Could you check a few things on this model? Use its own coordinates, in mm. A direction names the side the tool comes from. Round coordinates to 2 decimals unless told otherwise and drop trailing zeros. Loops run counter-clockwise (first coordinate to the right, second up) from the corner with the lowest first, then second, coordinate; pieces in that order, holes last. Notation, with made-up numbers: (-24, -33) - (-1, -33) arc R24 cw to (-1, -9) - close; hole circle Ø10 at (-18, 35). An arc over 180 degrees is marked (long way). Answer as CSV lines item,"result". Start each with the question number.
1) Which directions (+Z, -Z, +X, -X, +Y, -Y) give clear straight access to the entire face, cutting with the end or side of a thin tool? Please do faces 1 (the face through (25.5, 43, -63)), 2 (the face through (-20.5, -12, -58)), 3 (the face through (-28, -17.5, -10)), 4 (the face through (-30.3, 13.5, -17)).
2) We'd pull the mould along Z, two halves only. Please class faces 5 (the face through (0, 12, -34)), 6 (the face through (-6.5, 14, -34)), 7 (the face through (-21, 9, -14)): pulls with the +Z half, pulls with the -Z half, needs draft (parallel to the pull), parting line crosses it, or undercut.
3) Suppose I cut it at A-A, the plane z = -13. Write out the boundary of the cut face in (x, y), then the cut area to 3 significant figures.
4) Suppose I cut it at B-B, the plane x = 18.5. Write out the boundary of the cut face in (y, z).
5) Please list where these lines run through material, in increasing order: line 1 along X through (y, z) = (-1, -18.5); line 2 along Z through (x, y) = (-25.5, 3.5); line 3 along X through (y, z) = (42, -39).
6) Suppose I cut it at D-D, the plane y = 24. Write out the boundary of the cut face in (x, z), then the cut area to 3 significant figures.
7) Suppose I cut it at C-C, the plane x = -22. Write out the boundary of the cut face in (y, z).
8) I'm going to push flat-ended pins straight in: pin 1 Ø9.5 at (x, z) = (14.5, -46) entering from -Y; pin 2 Ø1.5 at (y, z) = (15, -32) entering from -X; pin 3 Ø3.5 at (y, z) = (-4, -5) entering from +X; pin 4 Ø24 at (y, z) = (20.5, -50.5) entering from -X. Where does each tip first touch, or does it pass through?
```python
from build123d import *

# Parameters (mm, degrees)
SKETCH1_W           = 69
SKETCH1_H           = 35
BOSS_EXTRUDE1_DEPTH = 68
CUT_EXTRUDE1_DEPTH  = 79.233624485
FILLET1_R           = 10
CUT_EXTRUDE2_DEPTH  = 14
CUT_EXTRUDE3_DEPTH  = 14
SKETCH6_W           = 18
SKETCH6_H           = 16
BOSS_EXTRUDE2_DEPTH = 33
CUT_EXTRUDE4_DEPTH  = 28
FILLET3_R           = 14
BOSS_EXTRUDE3_DEPTH = 9
FILLET4_R           = 14


with BuildPart() as part:
    # Sketch1 → Boss-Extrude1 (new body)
    with BuildSketch(Plane.XY):
        Rectangle(SKETCH1_W, SKETCH1_H)
    extrude(amount=-BOSS_EXTRUDE1_DEPTH)

    # Sketch2 → Cut-Extrude1 (cut, through all)
    with BuildSketch(Plane.XY):
        with BuildLine():
            Line((-20.5, -17.5), (-20.5, -7))
            Line((-20.5, -7), (-12, -7))
            Line((-12, -7), (-12, 0))
            ThreePointArc((-12, 0), (0, 12), (12, 0))
            Line((12, 0), (12, -7))
            Line((12, -7), (20.5, -7))
            Line((20.5, -7), (20.5, -17.5))
            Line((20.5, -17.5), (-20.5, -17.5))
        make_face()
    extrude(amount=-CUT_EXTRUDE1_DEPTH, mode=Mode.SUBTRACT)

    # Fillet1
    fillet1_edges = [part.edges().sort_by_distance(p)[0] for p in [
        (34.5, 0, 0),
        (-34.5, 0, 0),
    ]]
    fillet(fillet1_edges, radius=FILLET1_R)

    # Sketch4 → Cut-Extrude2 (cut)
    with BuildSketch(Plane.XY):
        Polygon((0, 17.5), (-34.5, -3.5), (-34.5, 17.5), align=None)
    extrude(amount=-CUT_EXTRUDE2_DEPTH, mode=Mode.SUBTRACT)

    # Sketch5 → Cut-Extrude3 (cut, symmetric)
    with BuildSketch(Plane.XY.offset(-34)):
        with BuildLine():
            Line((-34.5, -17.5), (-20.5, -17.5))
            Line((-20.5, -17.5), (-20.5, -10.5))
            Line((-20.5, -10.5), (-11.239870411, -10.5))
            Line((-11.239870411, -10.5), (-11.239870411, 0))
            ThreePointArc((-11.239870411, 0), (-10, 5.760129589), (-6.5, 10.5))
            Line((-6.5, 10.5), (-6.5, 17.5))
            Line((-6.5, 17.5), (-34.5, 17.5))
            Line((-34.5, 17.5), (-34.5, -17.5))
        make_face()
    extrude(amount=CUT_EXTRUDE3_DEPTH, both=True, mode=Mode.SUBTRACT)

    # Sketch6 → Boss-Extrude2 (add)
    with BuildSketch(Plane.XY.offset(-35)):
        with Locations((25.5, 25.5)):
            Rectangle(SKETCH6_W, SKETCH6_H)
    extrude(amount=-BOSS_EXTRUDE2_DEPTH)

    # Sketch7 → Cut-Extrude4 (cut)
    with BuildSketch(Plane.ZY.offset(-16.5)):
        with BuildLine():
            Line((-58, 33.5), (-58, 31.5))
            ThreePointArc((-58, 31.5), (-51.5, 25), (-45, 31.5))
            Line((-45, 31.5), (-45, 33.5))
            Line((-45, 33.5), (-58, 33.5))
        make_face()
    extrude(amount=-CUT_EXTRUDE4_DEPTH, mode=Mode.SUBTRACT)

    # Fillet3
    # the kernel refuses this fillet: 14 mm, written as the material it takes off along each edge
    with BuildSketch(Plane(origin=(-69.5, 17.5, -68), x_dir=(0, -1, 0), z_dir=(1, 0, 0))) as fillet3_piece_1:
        with BuildLine():
            CenterArc((FILLET3_R, -FILLET3_R), FILLET3_R, 90, 90)
            Line((0, -FILLET3_R), (0, 0))
            Line((0, 0), (FILLET3_R, 0))
        make_face()
    extrude(amount=86, mode=Mode.SUBTRACT)

    # Sketch9 → Boss-Extrude3 (add)
    with BuildSketch(Plane(origin=(34.5, 0, 0), x_dir=(0, 0, -1), z_dir=(1, 0, 0))):
        with BuildLine():
            Line((58, 33.5), (58, 51.5))
            ThreePointArc((58, 51.5), (65.071067812, 48.571067812), (68, 41.5))
            Line((68, 41.5), (68, 33.5))
            Line((68, 33.5), (58, 33.5))
        make_face()
        with BuildLine():
            Line((45, 33.5), (45, 51.5))
            ThreePointArc((45, 51.5), (37.928932188, 48.571067812), (35, 41.5))
            Line((35, 41.5), (35, 33.5))
            Line((35, 33.5), (45, 33.5))
        make_face()
    extrude(amount=-BOSS_EXTRUDE3_DEPTH)

    # Fillet4
    fillet4_edges = [part.edges().sort_by_distance(p)[0] for p in [
        (-34.5, 17.5, -17),
    ]]
    fillet(fillet4_edges, radius=FILLET4_R)


solid = part.part
```
Filled sheet:
1,face 1,"+Z, -Z, -X, +Y"
1,face 2,"+Z, -Z, -Y"
1,face 3,"+Z, -Z, +X, -X, -Y"
1,face 4,"+Z, -X, +Y"
2,face 5,"needs draft"
2,face 6,"undercut"
2,face 7,"pulls with the +Z half"
3,outline,"(-34.5, -17.5) - (-20.5, -17.5) - (-20.5, -7) - (-12, -7) - (-12, 0) arc R12 cw to (12, 0) - (12, -7) - (20.5, -7) - (20.5, -17.5) - (34.5, -17.5) - (34.5, 17.5) - (0, 17.5) - (-34.5, -3.5) - close"
3,area,"1,230 mm²"
4,outline,"(-7, -68) - (33.5, -68) - (33.5, -58) - (31.5, -58) arc R6.5 cw to (31.5, -45) - (33.5, -45) - (33.5, -35) - (17.5, -35) - (17.5, 0) - (-7, 0) - close"
5,line 1,"-34.5 to -12, 12 to 34.5"
5,line 2,"-68 to -48, -20 to -14"
5,line 3,"25.5 to 34.5"
6,outline,"(16.5, -68) - (34.5, -68) - (34.5, -35) - (16.5, -35) - close"
6,area,"594 mm²"
7,outline,"(-17.5, -68) - (3.5, -68) arc R14 ccw to (17.5, -54) - (17.5, -48) - (-17.5, -48) - close; (-17.5, -20) - (17.42, -20) - (17.42, -14) - (4.11, -14) - (4.11, 0) - (-17.5, 0) - close"
8,pin 1,"y = -7"
8,pin 2,"x = -6.5"
8,pin 3,"x = 33.96"
8,pin 4,"x = -34.5"
